Solid Edge part; units mm, degrees
sketch "Sketch1" plane through (60.3162, 0, 60.3162) normal (0, -1, 0) x (1, 0, 0)
  circle A0 centre (-60.3162, -60.3162) radius 7.5
extrude "Protrusion1" add sketch "Sketch1" against normal blind 60
hole "Bohrung_1" at (0, 0, 0) direction (0, 1, 0) diameter 3.242 depth 25 thread major 4 thread length 20
hole "Bohrung_2" at (0, 60, 0) direction (0, -1, 0) diameter 3.242 depth 25 thread major 4 thread length 20
properties material "Aluminium, 1060"
Can you work these out from the model? Positions are in its coordinate system, mm. A direction names the side the tool comes from. Give positions to 0.01 mm unless a question says otherwise; leave off trailing zeros. Loops run counter-clockwise (first coordinate to the right, second up) from the corner with the lowest first, then second, coordinate; pieces in that order, holes last. Notation, with made-up numbers: M -38,43.5 L 7,43.5 A34 ccw 7,73.5 Z; hole C -7.75,77 d4. An arc over 180 degrees is marked long. Answer in a Markdown table with one row per item.
1. Suppose I cut it at B-B on y = 9. Write out the boundary of the cut face in (x, z), plus the area to 3 significant figures.
Taken from the geometry:
| item | result |
|---|---|
| outline | C 0,0 d15; hole C 0,0 d3.24 |
| area | 168 mm² |
2. Which directions (+Z, -Z, +X, -X, +Y, -Y) give clear straight access to the entire face, cutting with the end or side of a thin tool? Please do faces 1 (the flat face through (0, 35, 0)), 2 (the flat face through (0, 25, 0)), 3 (the flat face through (2, 60, 0)).
Taken from the geometry:
| item | result |
|---|---|
| face 1 | +Y |
| face 2 | -Y |
| face 3 | +Z, -Z, +X, -X, +Y |
3. Suppose I cut it at A-A on x = 0. Write out the boundary of the cut face in (y, z), plus the area to 3 significant figures.
Taken from the geometry:
| item | result |
|---|---|
| outline | M 0,-7.5 L 60,-7.5 L 60,-1.62 L 35,-1.62 L 35,1.62 L 60,1.62 L 60,7.5 L 0,7.5 L 0,1.62 L 25,1.62 L 25,-1.62 L 0,-1.62 Z |
| area | 738 mm² |
4. Suppose I cut it at C-C on z = 0. Write out the boundary of the cut face in (x, y), plus the area to 3 significant figures.
Taken from the geometry:
| item | result |
|---|---|
| outline | M -7.5,0 L -1.62,0 L -1.62,25 L 1.62,25 L 1.62,0 L 7.5,0 L 7.5,60 L 1.62,60 L 1.62,35 L -1.62,35 L -1.62,60 L -7.5,60 Z |
| area | 738 mm² |
5. Suppose I cut it at D-D on y = 32.5. Write out the boundary of the cut face in (x, z).
Taken from the geometry:
| item | result |
|---|---|
| outline | C 0,0 d15 |
6. For pin 1 Ø1.9 at (x, z) = (0, 0) entering from +Y; pin 2 Ø6 at (y, z) = (42.5, -4.5) entering from -X; pin 3 Ø3.5 at (x, z) = (0, 0) entering from +Y; pin 4 Ø3 at (y, z) = (7.5, 3.5) entering from +X, each with a flat end and sliding along its axis, tell me the tip position at first contact or that it passes through.
Taken from the geometry:
| item | result |
|---|---|
| pin 1 | stops at y = 35 |
| pin 2 | stops at x = -7.35 |
| pin 3 | stops at y = 60 |
| pin 4 | stops at x = 7.23 |
7. If I drill on line 1 along Z through (x, y) = (0, 16); line 2 along X through (y, z) = (45.5, -0.25); line 3 along Y through (x, z) = (-1.5, -0.5), over which ranges is the centre line in solid material (lowest first)?
Taken from the geometry:
| item | result |
|---|---|
| line 1 | z = -7.5 to -1.62, 1.62 to 7.5 |
| line 2 | x = -7.5 to -1.6, 1.6 to 7.5 |
| line 3 | y = 25 to 35 |
8. Thinking about a two-plate mould opening in X: for faces 4 (the flat face through (2, 0, 0)), 5 (the cylindrical face through (-7.493, 29.58, 0.33)), 6 (the cylindrical face through (1.438, 12.675, -0.748)), which applies, released by +X, released by -X, zero draft, split by the parting line, or undercut?
Taken from the geometry:
| item | result |
|---|---|
| face 4 | zero draft |
| face 5 | split by the parting line |
| face 6 | undercut |
